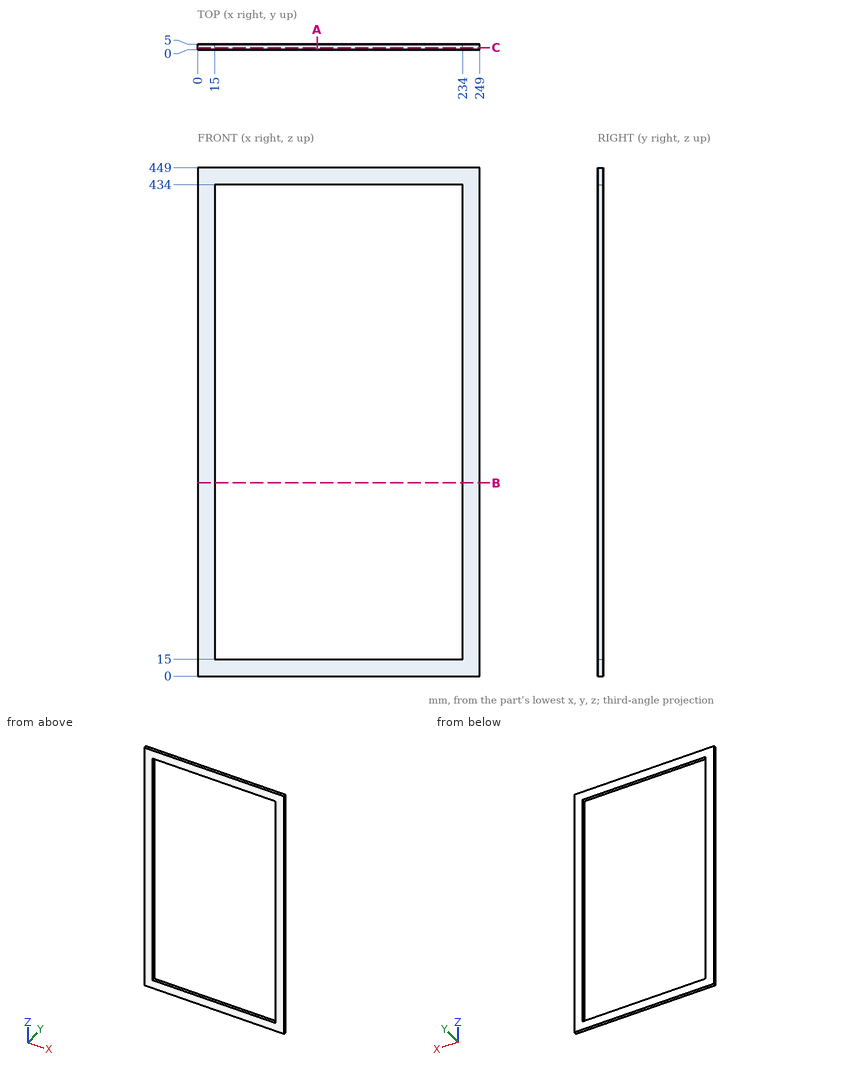
Can you work these out from the drawing? Everything is in mm from the part's minimum corner. Give positions to 0.01 mm unless a question says otherwise; leave off trailing zeros. Order: outer loops, then holes, each group sorted by start corner. A loop starts at its lowest first (then second) coordinate and runs counter-clockwise, first axis right, second up.
Item 1: If we section it at B-B, the plane z = 170.5: Write out the boundary of the cut face in (x, y).
Item 2: If we section it at A-A, the plane x = 105.5: Write out the boundary of the cut face in (y, z), plus the area to 3 significant figures.
Item 3: If we section it at C-C, the plane y = 1.75: Write out the boundary of the cut face in (x, z).
Item 4: I need wall thicknesses on line 1 (Z direction, x = 75, y = 0.5); line 2 (X direction, y = 3.95, z = 317). Which ranges of each line are inside material? Lowest first, please.
Values:
1. outline: (0, 0) - (15, 0) - (15, 5) - (0, 5) - close; (234, 0) - (249, 0) - (249, 5) - (234, 5) - close
2. outline: (0, 0) - (5, 0) - (5, 15) - (0, 15) - close; (0, 434) - (5, 434) - (5, 449) - (0, 449) - close
2. area: 150 mm2
3. outline: (0, 0) - (249, 0) - (249, 449) - (0, 449) - close; hole (15, 15) - (234, 15) - (234, 434) - (15, 434) - close
4. line 1: z = 0 to 15, 434 to 449
4. line 2: x = 0 to 15, 234 to 249
